```python
from build123d import *

# Parameters (mm, degrees)
SKETCH1_W           = 58
SKETCH1_H           = 30.5
BOSS_EXTRUDE1_DEPTH = 11.5
FILLET1_R           = 4.5
SKETCH2_W           = 9
SKETCH2_H           = 9
BOSS_EXTRUDE2_DEPTH = 2.4
FILLET2_R           = 1


with BuildPart() as part:
    # Sketch1 → Boss-Extrude1 (new body)
    with BuildSketch(Plane.XY):
        with Locations((29, 15.25)):
            Rectangle(SKETCH1_W, SKETCH1_H)
    extrude(amount=BOSS_EXTRUDE1_DEPTH)

    # Fillet1
    fillet1_edges = [part.edges().sort_by_distance(p)[0] for p in [
        (58, 15.25, 11.5),
        (0, 15.25, 11.5),
        (58, 15.25, 0),
        (0, 15.25, 0),
    ]]
    fillet(fillet1_edges, radius=FILLET1_R)

    # Sketch2 → Boss-Extrude2 (add)
    with BuildSketch(Plane(origin=(0, 30.5, 0), x_dir=(1, 0, 0), z_dir=(0, 1, 0))):
        with Locations((57.5, -5.75)):
            Rectangle(SKETCH2_W, SKETCH2_H)
    extrude(amount=BOSS_EXTRUDE2_DEPTH)

    # Fillet2
    fillet2_edges = [part.edges().sort_by_distance(p)[0] for p in [
        (0, 0, 5.75),
        (0, 30.5, 5.75),
        (29, 0, 0),
        (58, 0, 5.75),
        (29, 0, 11.5),
        (56.681980515, 0, 10.181980515),
        (56.681980515, 0, 1.318019485),
        (1.318019485, 0, 10.181980515),
        (1.318019485, 0, 1.318019485),
        (29, 30.5, 0),
        (29, 30.5, 11.5),
        (55.177050983, 30.5, 11.175823272),
        (1.318019485, 30.5, 10.181980515),
        (1.318019485, 30.5, 1.318019485),
        (55.177050983, 30.5, 0.324176728),
        (53, 30.5, 5.75),
        (53, 32.9, 5.75),
        (57.5, 32.9, 10.25),
        (57.5, 32.9, 1.25),
    ]]
    fillet(fillet2_edges, radius=FILLET2_R)


solid = part.part
```
Here's how the part is built. I have some questions about the finished solid (model axes, mm). A direction names the side the tool comes from. Coordinates: 2 decimals unless noted, no trailing zeros. Loops run counter-clockwise (first coordinate to the right, second up) from the corner with the lowest first, then second, coordinate; pieces in that order, holes last. Notation, with made-up numbers: (0.25, 29) - (37.25, 29) arc R21 ccw to (37.25, 54) - close; hole circle Ø11 at (58.25, 31). An arc over 180 degrees is marked (long way). Answer as CSV lines item,"result".
Q1. If we section it at B-B, the plane y = 18: Write out the boundary of the cut face in (x, z), and give its area (3 significant figures).
Response:
outline,"(0, 4.5) arc R4.5 ccw to (4.5, 0) - (53.5, 0) arc R4.5 ccw to (58, 4.5) - (58, 7) arc R4.5 ccw to (53.5, 11.5) - (4.5, 11.5) arc R4.5 ccw to (0, 7) - close"
area,"650 mm2"
Q2. If I drill on L1, parallel to X at y = 12.5, z = 4.75; L2, parallel to Y at x = 9, z = 5.5; L3, parallel to Y at x = 53.5, z = 7, over which ranges is the centre line in solid material (lowest first)? Write a range as [from, to].
Response:
L1,"[0, 58]"
L2,"[0, 30.5]"
L3,"[0, 32.77]"
Q3. If we section it at A-A, the plane x = 30: Write out the boundary of the cut face in (y, z).
Response:
outline,"(0, 1) arc R1 ccw to (1, 0) - (29.5, 0) arc R1 ccw to (30.5, 1) - (30.5, 10.5) arc R1 ccw to (29.5, 11.5) - (1, 11.5) arc R1 ccw to (0, 10.5) - close"
Q4. For pin 1 (4.5 mm diameter, centred on x = 59.5, z = 6.5, fed in from -Y); pin 2 (1.9 mm diameter, centred on x = 59, y = 30, fed in from -Z); pin 3 (1.3 mm diameter, centred on y = 13, z = 5.5, fed in from +X), each with a flat end and sliding along its axis, tell me the tip position at first contact or that it passes through.
Response:
pin 1,"y = 0.03"
pin 2,"z = 1.25"
pin 3,"x = 58"
Q5. For faces 1 (the face through (56.717, 15.956, 10.147)), 2 (the face through (56.717, 15.956, 1.353)), 3 (the face through (58, 32.9, 6)), 4 (the face through (29, 0, 6)), 5 (the face through (58, 16, 6)), which set-ups out of +Z, -Z, +X, -X, +Y, -Y let a thin tool reach every point of the face, with its end or its side?
Response:
face 1,"+Z, +X, -Y"
face 2,"-Z, +X, -Y"
face 3,"+Z, -Z, +X, -X, +Y"
face 4,"+Z, -Z, +X, -X, -Y"
face 5,"+Z, -Z, +X, -Y"
